Check sheet for the drawn part. Datum: minimum x, y, z corner. Units: mm. Round coordinates to 2 decimals unless told otherwise and drop trailing zeros. Write each loop counter-clockwise with the first axis right and the second up, starting at its lowest first coordinate (ties: lowest second). Pieces come first, ordered by that corner, then holes. Notation, with made-up numbers: M 4.5,12 L 53.5,12 A26 ccw 53.5,42 Z; hole C 84.25,-6.5 d11. An arc over 180 degrees is marked long. One line per item, written item: value. Start each with the question number.
Item 1: Thickness scan on probe 1 along Z at (x, y) = (8, 12.5); probe 2 along Z at (x, y) = (8, 5.75); probe 3 along X at (y, z) = (5.75, 7). Record the ranges inside material, lowest first. Write a range as from..to.
Item 2: Section check C-C, the plane z = 150. Record the cut outline in (x, y), then the cut area to 3 significant figures.
Item 3: Section check A-A, the plane x = 8. Record the cut outline in (y, z).
Item 4: Section check D-D, the plane x = 1.5. Record the cut outline in (y, z).
Item 5: Gauge pin test, flat ends, axial feed: pin 1 (6 mm diameter, centred on y = 2, z = 132, fed in from +X); pin 2 (3 mm diameter, centred on y = 11.5, z = 60.5, fed in from +X); pin 3 (3 mm diameter, centred on y = 14, z = 108, fed in from +X). Record the tip position at first contact, or that the pin passes through.
Item 6: Section check B-B, the plane z = 29.5. Record the cut outline in (x, y).
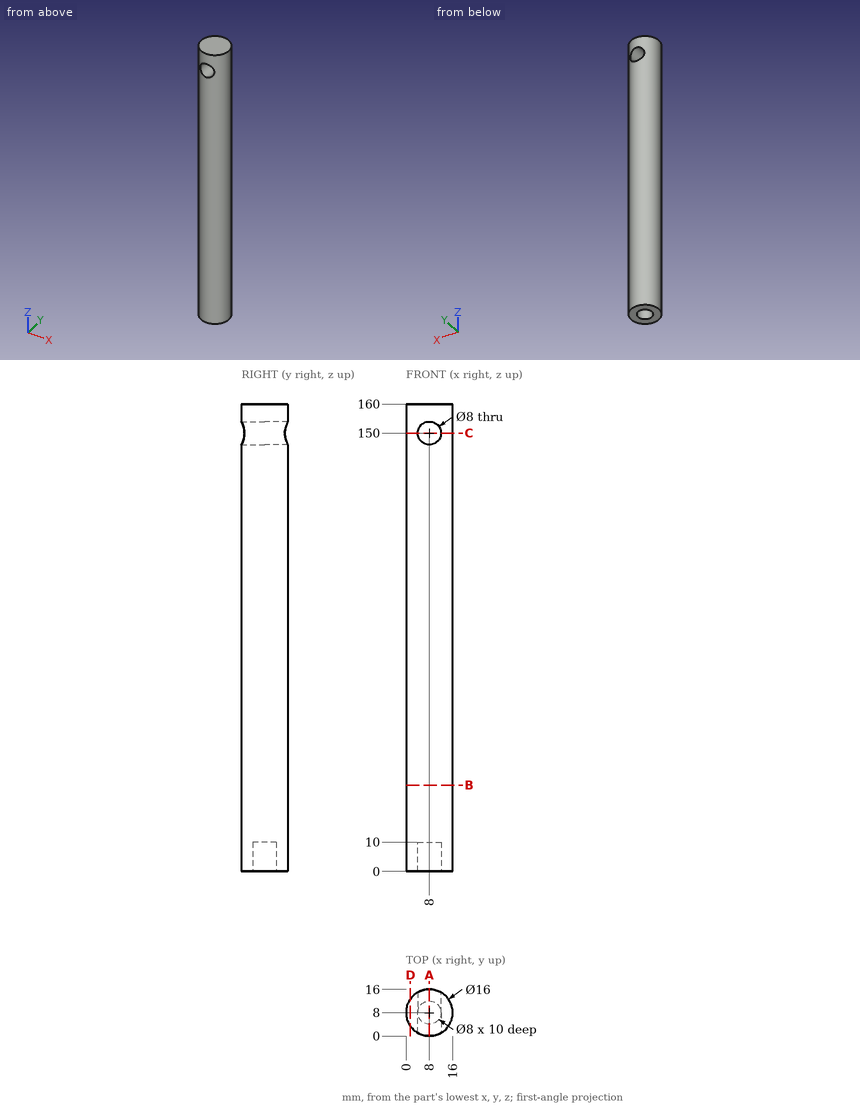
Response values:
1. probe 1: z = 0..146, 154..160
1. probe 2: z = 10..146, 154..160
1. probe 3: x = 0.32..4.69, 11.31..15.68
2. outline: M 4,1.07 L 4,14.93 A8 ccw Z; M 12,1.07 A8 ccw 12,14.93 Z
2. area: 78.6 mm2
3. outline: M 0,0 L 4,0 L 4,10 L 12,10 L 12,0 L 16,0 L 16,146 L 0,146 Z; M 0,154 L 16,154 L 16,160 L 0,160 Z
4. outline: M 3.34,0 L 12.66,0 L 12.66,160 L 3.34,160 Z
5. pin 1: stops at x = 15.42
5. pin 2: stops at x = 15.75
5. pin 3: stops at x = 14.61
6. outline: C 8,8 d16
